```python
from build123d import *

# Parameters (mm, degrees)
BOSS_EXTRUDE1_DEPTH     = 6.5
SKETCH2_R               = 21.5
BOSS_EXTRUDE2_DEPTH     = 2.5
CUT_EXTRUDE1_DEPTH      = 8
SKETCH4_W               = 3
SKETCH4_H               = 3
CUT_EXTRUDE2_DEPTH      = 10
SKETCH5_R               = 5
BOSS_EXTRUDE3_DEPTH     = 140
CUT_EXTRUDE3_DEPTH      = 15
MIRROR6_COPY_1_SKETCH_R = 21.5
MIRROR6_COPY_1_DEPTH    = 2.5
MIRROR6_COPY_2_SKETCH_W = 3
MIRROR6_COPY_2_SKETCH_H = 3
MIRROR6_COPY_2_DEPTH    = 10


with BuildPart() as part:
    # Sketch1 → Boss-Extrude1 (new body)
    with BuildSketch(Plane(origin=(0, 0, 0), x_dir=(1, 0, 0), z_dir=(0, 1, 0))):
        with BuildLine():
            ThreePointArc((-1.9, -2.05669638), (-2.8, 0), (-1.9, 2.05669638))
            Line((-1.9, 2.05669638), (-1.9, 5.532856405))
            ThreePointArc((-1.9, 5.532856405), (-5.85, 0), (-1.9, -5.532856405))
            Line((-1.9, -5.532856405), (-1.9, -2.05669638))
        make_face()
        with BuildLine():
            ThreePointArc((-1.9, 2.05669638), (0, 2.8), (1.9, 2.05669638))
            Line((1.9, 2.05669638), (1.9, 5.532856405))
            ThreePointArc((1.9, 5.532856405), (0, 5.85), (-1.9, 5.532856405))
            Line((-1.9, 5.532856405), (-1.9, 2.05669638))
        make_face()
        with BuildLine():
            Line((1.9, 5.532856405), (1.9, 2.05669638))
            ThreePointArc((1.9, 2.05669638), (2.565151068, 1.122497216), (2.8, 0))
            ThreePointArc((2.8, 0), (2.565151068, -1.122497216), (1.9, -2.05669638))
            Line((1.9, -2.05669638), (1.9, -5.532856405))
            ThreePointArc((1.9, -5.532856405), (4.761171074, -3.399080758), (5.85, 0))
            ThreePointArc((5.85, 0), (4.761171074, 3.399080758), (1.9, 5.532856405))
        make_face()
        with BuildLine():
            Line((1.9, -5.532856405), (1.9, -2.05669638))
            ThreePointArc((1.9, -2.05669638), (0, -2.8), (-1.9, -2.05669638))
            Line((-1.9, -2.05669638), (-1.9, -5.532856405))
            ThreePointArc((-1.9, -5.532856405), (0, -5.85), (1.9, -5.532856405))
        make_face()
        with BuildLine():
            Line((-1.9, -2.05669638), (-1.9, 2.05669638))
            ThreePointArc((-1.9, 2.05669638), (-2.8, 0), (-1.9, -2.05669638))
        make_face()
        with BuildLine():
            ThreePointArc((2.8, 0), (2.565151068, 1.122497216), (1.9, 2.05669638))
            Line((1.9, 2.05669638), (1.9, -2.05669638))
            ThreePointArc((1.9, -2.05669638), (2.565151068, -1.122497216), (2.8, 0))
        make_face()
    boss_extrude1 = extrude(amount=BOSS_EXTRUDE1_DEPTH)

    # Sketch2 → Boss-Extrude2 (add)
    with BuildSketch(Plane(origin=(0, 6.5, 0), x_dir=(1, 0, 0), z_dir=(0, 1, 0))):
        with Locations(Location((0, 0, 0), (0, 0, 270))):
            Circle(SKETCH2_R)
    boss_extrude2 = extrude(amount=-BOSS_EXTRUDE2_DEPTH)

    # Sketch3 → Cut-Extrude1 (cut)
    with BuildSketch(Plane.XZ.offset(-4)):
        with BuildLine():
            Line((-1.9, 2.05669638), (-1.9, -2.05669638))
            ThreePointArc((-1.9, -2.05669638), (0, -2.8), (1.9, -2.05669638))
            Line((1.9, -2.05669638), (1.9, 2.05669638))
            ThreePointArc((1.9, 2.05669638), (0, 2.8), (-1.9, 2.05669638))
        make_face()
    cut_extrude1 = extrude(amount=-CUT_EXTRUDE1_DEPTH, mode=Mode.SUBTRACT)

    # Sketch4 → Cut-Extrude2 (cut)
    with BuildSketch(Plane(origin=(0, 6.5, 0), x_dir=(1, 0, 0), z_dir=(0, 1, 0))):
        Polygon((15.202795796, -13.081475452), (17.324116139, -15.202795796), (15.202795796, -17.324116139), (13.081475452, -15.202795796), align=None)
        with Locations((21.5, 0)):
            Rectangle(SKETCH4_W, SKETCH4_H)
        with Locations((0, -21.5)):
            Rectangle(SKETCH4_W, SKETCH4_H)
        Polygon((-13.081475452, -15.202795796), (-15.202795796, -17.324116139), (-17.324116139, -15.202795796), (-15.202795796, -13.081475452), align=None)
        with Locations((-21.5, 0)):
            Rectangle(SKETCH4_W, SKETCH4_H)
        Polygon((-15.202795796, 13.081475452), (-17.324116139, 15.202795796), (-15.202795796, 17.324116139), (-13.081475452, 15.202795796), align=None)
        with Locations((0, 21.5)):
            Rectangle(SKETCH4_W, SKETCH4_H)
        Polygon((13.081475452, 15.202795796), (15.202795796, 17.324116139), (17.324116139, 15.202795796), (15.202795796, 13.081475452), align=None)
    cut_extrude2 = extrude(amount=-CUT_EXTRUDE2_DEPTH, mode=Mode.SUBTRACT)

    # Sketch5 → Boss-Extrude3 (add)
    with BuildSketch(Plane(origin=(0, 6.5, 0), x_dir=(1, 0, 0), z_dir=(0, 1, 0))):
        with Locations(Location((0, 0, 0), (0, 0, 270))):
            Circle(SKETCH5_R)
    extrude(amount=BOSS_EXTRUDE3_DEPTH)

    # Mirror1: Boss-Extrude2 across plane
    add(boss_extrude2.mirror(Plane.ZX.offset(76.5)))

    # Mirror2: Boss-Extrude1 across plane
    add(boss_extrude1.mirror(Plane.ZX.offset(76.5)))

    # Mirror3: Boss-Extrude2, Cut-Extrude1, Cut-Extrude2 across plane
    add(boss_extrude2.mirror(Plane.ZX.offset(7.5)))
    add(cut_extrude1.mirror(Plane.ZX.offset(7.5)), mode=Mode.SUBTRACT)
    add(cut_extrude2.mirror(Plane.ZX.offset(7.5)), mode=Mode.SUBTRACT)

    # Sketch6 → Cut-Extrude3 (cut)
    with BuildSketch(Plane.XZ.offset(-11)):
        with BuildLine():
            Line((-1.9, 2.05669638), (-1.9, -2.05669638))
            ThreePointArc((-1.9, -2.05669638), (0, -2.8), (1.9, -2.05669638))
            Line((1.9, -2.05669638), (1.9, 2.05669638))
            ThreePointArc((1.9, 2.05669638), (0, 2.8), (-1.9, 2.05669638))
        make_face()
    extrude(amount=-CUT_EXTRUDE3_DEPTH, mode=Mode.SUBTRACT)

    # Mirror5: Cut-Extrude2 across plane
    add(cut_extrude2.mirror(Plane.ZX.offset(76.5)), mode=Mode.SUBTRACT)

    # Mirror6 copy 1 sketch → Mirror6 copy 1 (add)
    with BuildSketch(Plane(origin=(0, 144.5, 0), x_dir=(1, 0, 0), z_dir=(0, 1, 0))):
        with Locations(Location((0, 0, 0), (0, 0, 270))):
            Circle(MIRROR6_COPY_1_SKETCH_R)
    extrude(amount=-MIRROR6_COPY_1_DEPTH)

    # Mirror6 copy 2 sketch → Mirror6 copy 2 (cut)
    with BuildSketch(Plane(origin=(0, 144.5, 0), x_dir=(1, 0, 0), z_dir=(0, 1, 0))):
        Polygon((15.202795796, -13.081475452), (17.324116139, -15.202795796), (15.202795796, -17.324116139), (13.081475452, -15.202795796), align=None)
        with Locations((21.5, 0)):
            Rectangle(MIRROR6_COPY_2_SKETCH_W, MIRROR6_COPY_2_SKETCH_H)
        with Locations((0, -21.5)):
            Rectangle(MIRROR6_COPY_2_SKETCH_W, MIRROR6_COPY_2_SKETCH_H)
        Polygon((-13.081475452, -15.202795796), (-15.202795796, -17.324116139), (-17.324116139, -15.202795796), (-15.202795796, -13.081475452), align=None)
        with Locations((-21.5, 0)):
            Rectangle(MIRROR6_COPY_2_SKETCH_W, MIRROR6_COPY_2_SKETCH_H)
        Polygon((-15.202795796, 13.081475452), (-17.324116139, 15.202795796), (-15.202795796, 17.324116139), (-13.081475452, 15.202795796), align=None)
        with Locations((0, 21.5)):
            Rectangle(MIRROR6_COPY_2_SKETCH_W, MIRROR6_COPY_2_SKETCH_H)
        Polygon((13.081475452, 15.202795796), (15.202795796, 17.324116139), (17.324116139, 15.202795796), (15.202795796, 13.081475452), align=None)
    extrude(amount=-MIRROR6_COPY_2_DEPTH, mode=Mode.SUBTRACT)


solid = part.part
```
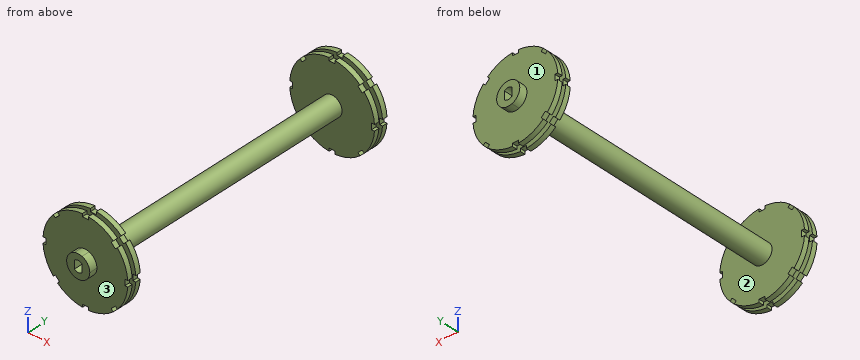
Can you work these out from the model? Positions are in its coordinate system, mm. Face numbers are marked on the shaded views. Round coordinates to 2 decimals unless told otherwise and drop trailing zeros. Order: outer loops, then holes, each group sorted by start corner. A loop starts at its lowest first (then second) coordinate and runs counter-clockwise, first axis right, second up. Notation, with made-up numbers: (47, -10) -> (91, -10) arc R19 ccw to (91, -6) -> close; hole circle Ø4 at (-32.5, 84.5). An arc over 180 degrees is marked (long way). Return JSON: item names as keys, results as strings. Group by question number.
1. If we section it at A-A, the plane y = 13: Write out the boundary of the cut face in (x, z), then the cut area to 3 significant figures.
2. If we section it at B-B, the plane x = -10.5: Write out the boundary of the cut face in (y, z), then the cut area to 3 significant figures.
3. We'd pull the mould along Y, two halves only. Please class the marked faces 1, 2 and 3: released by +Y, released by -Y, zero draft, split by the parting line, or undercut.
4. If we section it at C-C, the plane y = 116: Write out the boundary of the cut face in (x, z).
5. Will these pins go through, and if not, where does the flat tip stop? pin 1 (1.2 mm diameter, centred on y = 147, z = 20.5, fed in from -X); pin 2 (1.6 mm diameter, centred on y = 10, z = -20.5, fed in from +X); pin 3 (1.6 mm diameter, centred on x = 20.5, y = 10, fed in from -Z).
6. I need wall thicknesses on line 1 (Y direction, x = -2.5, z = -14.5); line 2 (X direction, y = 142.5, z = -13); line 3 (X direction, y = 9.5, z = 16). Which ranges of each line are inside material? Lowest first, please. Write a range as [from, to].
Output values:
{
 "1": {"outline": "circle Ø10 at (0, 0); hole (-1.9, -2.06) arc R2.8 ccw to (1.9, -2.06) -> (1.9, 2.06) arc R2.8 ccw to (-1.9, 2.06) -> close", "area": "59.0 mm²"},
 "2": {"outline": "(4, -18.76) -> (6.5, -18.76) -> (6.5, 18.76) -> (4, 18.76) -> close; (8.5, -18.76) -> (11, -18.76) -> (11, 18.76) -> (8.5, 18.76) -> close; (142, -18.76) -> (144.5, -18.76) -> (144.5, 18.76) -> (142, 18.76) -> close; (146.5, -18.76) -> (149, -18.76) -> (149, 18.76) -> (146.5, 18.76) -> close", "area": "375 mm²"},
 "3": {"face 1": "released by +Y", "face 2": "undercut", "face 3": "released by -Y"},
 "4": {"outline": "circle Ø10 at (0, 0)"},
 "5": {"pin 1": "x = -8.14", "pin 2": "x = 8.61", "pin 3": "z = -8.61"},
 "6": {"line 1": "[4, 6.5], [8.5, 11], [142, 144.5], [146.5, 149]", "line 2": "[-17.12, 17.12]", "line 3": "[-13.88, 13.88]"}
}
